Read the model definition and answer for the solid it produces. Units are mm, in the model's axes. A direction names the side the tool comes from. Coordinates: 2 decimals unless noted, no trailing zeros. Loops run counter-clockwise (first coordinate to the right, second up) from the corner with the lowest first, then second, coordinate; pieces in that order, holes last. Notation, with made-up numbers: M 34.25,62 L 46.25,62 A12 cw 46.25,70 Z; hole C 43,10 d9. An arc over 180 degrees is marked long. Use one line per item in the form item = value. Start each with the question number.
1. For a pull along Y with two mould halves and no side action, classify faces 3 (the cylindrical face through (2.67, -6.47, 2.97)), 4 (the conical face through (-0.031, 5.961, 0.618)), 5 (the cylindrical face through (-0.585, -2.636, 4.521)) as released by +Y, released by -Y, zero draft, split by the parting line, or undercut.
2. Find the intervals of material crossed by probe 1 along Y at (x, z) = (0, 5.35); probe 2 along Z at (x, y) = (-5.25, -2); probe 3 along Z at (x, y) = (-2, 0.25), in increasing order. Write a range as [from, to].
3. A tool of negligible diameter and unlimited length cuts with its end or side. For faces 1 (the conical face through (-4.19, -4.24, 0.62)), 2 (the flat face through (0, 0, 3)), from which of +Z, -Z, +X, -X, +Y, -Y can it reach the whole face along a straight path? Write none if from no direction.
4. The part is cut by section D-D (z = 0.75). Give the vertices of the cut face in (x, y).
5. Flat-ended cylindrical pins translate along their axes: pin 1 (1.5 mm diameter, centred on x = 4, y = -4.5, fed in from +Z); pin 2 (2.5 mm diameter, centred on x = 1, y = 1, fed in from +Z). Find the tip coordinate at first contact, or state that the pin passes through.
6. The part is cut by section A-A (z = 4). Give the vertices of the cut face in (x, y), plus the area to 3 significant figures.
7. The part is cut by section B-B (y = 0). Give the vertices of the cut face in (x, z).
from build123d import *

# Parameters (mm, degrees)
ESQUISSE1_R                  = 7
BOSS_EXTRU_1_DEPTH           = 5
ENL_V_MAT_EXTRU_2_DEPTH      = 6
R_P_TITION_CIRCULAIRE1_COUNT = 8
CHANFREIN1_SIZE              = 1
ESQUISSE3_R                  = 4
BOSS_EXTRU_2_DEPTH           = 1
ESQUISSE4_R                  = 2.7
ENL_V_MAT_EXTRU_3_DEPTH      = 3


with BuildPart() as part:
    # Esquisse1 → Boss.-Extru.1 (new body)
    with BuildSketch(Plane.XY):
        Circle(ESQUISSE1_R)
    extrude(amount=BOSS_EXTRU_1_DEPTH)

    # Esquisse2 → Enlèv. mat.-Extru.2 (cut, through all)
    with BuildSketch(Plane.XY.offset(5)):
        with BuildLine():
            ThreePointArc((2, 6.708203932), (0, 6.342871257), (-2, 6.708203932))
            ThreePointArc((-2, 6.708203932), (0, 7), (2, 6.708203932))
        make_face()
    enl_v_mat_extru_2 = extrude(amount=-ENL_V_MAT_EXTRU_2_DEPTH, mode=Mode.SUBTRACT)

    # Répétition circulaire1: Enlèv. mat.-Extru.2 ×8 about axis
    r_p_tition_circulaire1_axis = Axis((0, 0, 0), (0, 0, 1))
    for i in range(1, R_P_TITION_CIRCULAIRE1_COUNT):
        add(enl_v_mat_extru_2.rotate(r_p_tition_circulaire1_axis, i * 360 / R_P_TITION_CIRCULAIRE1_COUNT), mode=Mode.SUBTRACT)

    # Chanfrein1
    chanfrein1_edges = [part.edges().sort_by_distance(p)[0] for p in [
        (-6.467156728, 2.678784027, 0),
        (-6.467156728, -2.678784027, 0),
        (-2.678784027, -6.467156728, 0),
        (2.678784027, -6.467156728, 0),
        (6.467156728, -2.678784027, 0),
        (6.467156728, 2.678784027, 0),
        (2.678784027, 6.467156728, 0),
        (-6.342871257, 0, 0),
        (-4.485087278, -4.485087278, 0),
        (0, -6.342871257, 0),
        (4.485087278, -4.485087278, 0),
        (6.342871257, 0, 0),
        (4.485087278, 4.485087278, 0),
        (-2.678784027, 6.467156728, 0),
        (-4.485087278, 4.485087278, 0),
        (0, 6.342871257, 0),
    ]]
    chamfer(chanfrein1_edges, length=CHANFREIN1_SIZE)

    # Esquisse3 → Boss.-Extru.2 (add)
    with BuildSketch(Plane.XY.offset(5)):
        Circle(ESQUISSE3_R)
    extrude(amount=BOSS_EXTRU_2_DEPTH)

    # Esquisse4 → Enlèv. mat.-Extru.3 (cut)
    with BuildSketch(Plane.XY.offset(6)):
        Circle(ESQUISSE4_R)
    extrude(amount=-ENL_V_MAT_EXTRU_3_DEPTH, mode=Mode.SUBTRACT)


solid = part.part
Computed values:
q1.face_3 = released by -Y
q1.face_4 = released by +Y
q1.face_5 = undercut
q2.probe_1 = [-4, -2.7], [2.7, 4]
q2.probe_2 = [0, 5]
q2.probe_3 = [0, 3]
q3.face_1 = -Z, -X, -Y
q3.face_2 = +Z
q4.outline = M -6.44,-2.01 A6.75 ccw -5.98,-3.14 A5.91 cw -3.14,-5.98 A6.75 ccw -2.01,-6.44 A5.91 cw 2.01,-6.44 A6.75 ccw 3.14,-5.98 A5.91 cw 5.98,-3.14 A6.75 ccw 6.44,-2.01 A5.91 cw 6.44,2.01 A6.75 ccw 5.98,3.14 A5.91 cw 3.14,5.98 A6.75 ccw 2.01,6.44 A5.91 cw -2.01,6.44 A6.75 ccw -3.14,5.98 A5.91 cw -5.98,3.14 A6.75 ccw -6.44,2.01 A5.91 cw Z
q5.pin_1 = 5
q5.pin_2 = 3
q6.outline = M -6.71,-2 A7 ccw -6.16,-3.33 A5.66 cw -3.33,-6.16 A7 ccw -2,-6.71 A5.66 cw 2,-6.71 A7 ccw 3.33,-6.16 A5.66 cw 6.16,-3.33 A7 ccw 6.71,-2 A5.66 cw 6.71,2 A7 ccw 6.16,3.33 A5.66 cw 3.33,6.16 A7 ccw 2,6.71 A5.66 cw -2,6.71 A7 ccw -3.33,6.16 A5.66 cw -6.16,3.33 A7 ccw -6.71,2 A5.66 cw Z; hole C 0,0 d5.4
q6.area = 117 mm²
q7.outline = M -6.34,1 L -5.34,0 L 5.34,0 L 6.34,1 L 6.34,5 L 4,5 L 4,6 L 2.7,6 L 2.7,3 L -2.7,3 L -2.7,6 L -4,6 L -4,5 L -6.34,5 Z
